```python
from build123d import *

# Parameters (mm, degrees)
BOSS_EXTRUDE1_START = -9
SKETCH2_R           = 7.5
BOSS_EXTRUDE1_DEPTH = 5
BOSS_EXTRUDE2_START = -4
BOSS_EXTRUDE2_DEPTH = 4
CUT_EXTRUDE1_START  = 4
SKETCH4_W           = 25
SKETCH4_H           = 10
CUT_EXTRUDE1_DEPTH  = 5


with BuildPart() as part:
    # Sketch2 → Boss-Extrude1 (new body)
    with BuildSketch(Plane(origin=(0, 0, 0), x_dir=(0, 0, -1), z_dir=(1, 0, 0)).offset(BOSS_EXTRUDE1_START)):
        with BuildLine():
            Line((-20, 0), (-20, -252))
            Line((-20, -252), (20, -252))
            Line((20, -252), (20, 0))
            ThreePointArc((20, 0), (0, 20), (-20, 0))
        make_face()
        Circle(SKETCH2_R, mode=Mode.SUBTRACT)
    extrude(amount=BOSS_EXTRUDE1_DEPTH)

    # Sketch2<6> → Boss-Extrude2 (add)
    with BuildSketch(Plane(origin=(0, 0, 0), x_dir=(0, 0, -1), z_dir=(1, 0, 0)).offset(BOSS_EXTRUDE2_START)):
        with BuildLine():
            Line((-20, 0), (-20, -252))
            Line((-20, -252), (20, -252))
            Line((20, -252), (20, 0))
            ThreePointArc((20, 0), (0, 20), (-20, 0))
        make_face()
        with BuildLine():
            Line((-15, 0), (-15, -247))
            Line((-15, -247), (15, -247))
            Line((15, -247), (15, 0))
            ThreePointArc((15, 0), (0, 15), (-15, 0))
        make_face(mode=Mode.SUBTRACT)
    extrude(amount=BOSS_EXTRUDE2_DEPTH)

    # Mirror1: part across plane


with BuildPart() as part_1:
    add(part.part)
    add(part.part.mirror(Plane(origin=(0, 0, 0), x_dir=(0, 0, 1), z_dir=(1, 0, 0))))

    # Sketch4 → Cut-Extrude1 (cut)
    with BuildSketch(Plane(origin=(0, 0, 0), x_dir=(0, 0, -1), z_dir=(1, 0, 0)).offset(CUT_EXTRUDE1_START)):
        with Locations((0, -100)):
            Rectangle(SKETCH4_W, SKETCH4_H)
    extrude(amount=CUT_EXTRUDE1_DEPTH, mode=Mode.SUBTRACT)


solid = part_1.part
```
Here's how the part is built. I have some questions about the finished solid (model axes, mm). A direction names the side the tool comes from. Coordinates: 2 decimals unless noted, no trailing zeros. Order: outer loops, then holes, each group sorted by start corner. A loop starts at its lowest first (then second) coordinate and runs counter-clockwise, first axis right, second up. Notation, with made-up numbers: (-30.75, -4) -> (-12.75, -4) arc R32 cw to (-12.75, 22) -> close; hole circle Ø5 at (71, -40). An arc over 180 degrees is marked (long way). Return JSON: item names as keys, results as strings.
1) I'm going to push flat-ended pins straight in: P1, Ø4, axis at x = -1.5, z = -3, coming from the +Y side (3 decimals); P2, Ø6, axis at x = -6, z = -6.5, coming from the +Y side; P3, Ø1.5, axis at x = 6.5, z = -5.5, coming from the +Y side. Where does each tip first touch, or does it pass through?
Conclusion:
{"P1": "stops at y = 19.975", "P2": "stops at y = 19.69", "P3": "stops at y = 19.43"}
2) On a 3-axis mill with a long thin cutter (end or side, diameter ignored), from which of +Z, -Z, +X, -X, +Y, -Y can I reach the whole of each face in a straight line? I mean faces 1 (the cylindrical face through (0, 15, 0)), 2 (the cylindrical face through (-6.535, 0.33, 7.493)), 3 (the flat face through (6, -105, 0)). Say none if no direction works.
Conclusion:
{"face 1": "none", "face 2": "+X, -X", "face 3": "+X"}
3) Thinking about a two-plate mould opening in Y: for faces 4 (the flat face through (0, -252, 0)), 5 (the flat face through (-9, -114, 0)), 6 (the flat face through (-4, -114, 0)), which applies, +Y half, -Y half, draft (parallel to the pull), parting line (faces both ways), or undercut?
Conclusion:
{"face 4": "-Y half", "face 5": "draft", "face 6": "undercut"}
4) If we section it at C-C on x = 1.5: List the corners of the cut face in (y, z) for me, plus the area to 3 significant figures.
Conclusion:
{"outline": "(-252, -20) -> (0, -20) arc R20 ccw to (0, 20) -> (-252, 20) -> close; hole (-247, -15) -> (0, -15) arc R15 ccw to (0, 15) -> (-247, 15) -> close", "area": "2,940 mm²"}
5) If we section it at A-A on y = -10.5: List the corners of the cut face in (x, z) for me.
Conclusion:
{"outline": "(-9, -20) -> (9, -20) -> (9, 20) -> (-9, 20) -> close; hole (-4, -15) -> (4, -15) -> (4, 15) -> (-4, 15) -> close"}
6) If we section it at B-B on z = 0: List the corners of the cut face in (x, y) for me.
Conclusion:
{"outline": "(-9, -252) -> (9, -252) -> (9, -105) -> (4, -105) -> (4, -247) -> (-4, -247) -> (-4, -7.5) -> (-9, -7.5) -> close; (-9, 7.5) -> (-4, 7.5) -> (-4, 15) -> (4, 15) -> (4, 7.5) -> (9, 7.5) -> (9, 20) -> (-9, 20) -> close; (4, -95) -> (9, -95) -> (9, -7.5) -> (4, -7.5) -> close"}
7) If I drill on probe 1 along Y at (x, z) = (7.9, 0); probe 2 along X at (y, z) = (-83, 12); probe 3 along Z at (x, y) = (-3, -97), over which ranges is the centre line in solid material (lowest first)?
Conclusion:
{"probe 1": "y = -252 to -105, -95 to -7.5, 7.5 to 20", "probe 2": "x = -9 to -4, 4 to 9", "probe 3": "z = -20 to -15, 15 to 20"}
